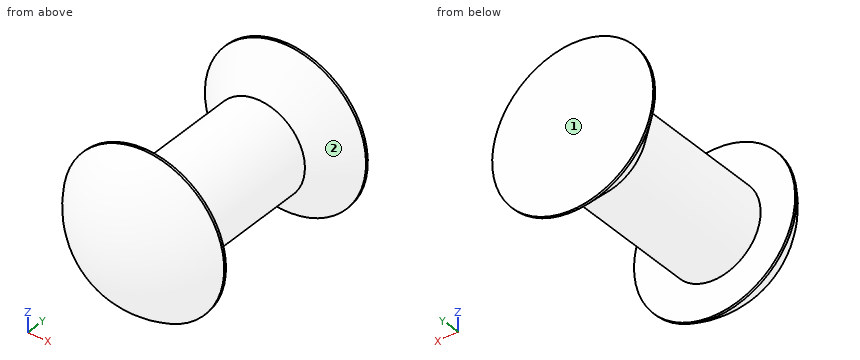
from build123d import *

# Parameters (mm, degrees)
EXTRUDE_1_DEPTH      = 0.4
EXTRUDE_1_DEPTH_BACK = 2
SKETCH_2_R           = 2
SKETCH_3_R           = 3.5
EXTRUDE_2_DEPTH      = 0.1
DOME_1_FACE_RADIUS   = 3.5
DOME_1_HEIGHT        = 2


with BuildPart() as part:
    # Эскиз1 → Revolve 344 (revolve)
    with BuildSketch(Plane.XY, mode=Mode.PRIVATE) as revolve_344_sk:
        with BuildLine():
            Line((0, 0), (1.6, 0))
            ThreePointArc((1.6, 0), (1.882842712, 0.117157288), (2, 0.4))
            Line((2, 0.4), (2, 6))
            Line((2, 6), (3.5, 7.5))
            Line((3.5, 7.5), (3.5, 7.6))
            Line((3.5, 7.6), (0, 7.6))
            Line((0, 7.6), (0, 0))
        make_face()
    revolve(revolve_344_sk.sketch.rotate(Axis((0, 11.283972125, 0), (0, -1, 0)), 90), axis=Axis((0, 11.283972125, 0), (0, -1, 0)))

    # Эскиз2 → Вытянуть1 (add, two sides: drawn at the far end of the back side and taken through both)
    with BuildSketch(Plane.XZ.offset(-EXTRUDE_1_DEPTH_BACK)):
        with Locations(Location((0, 0, 0), (0, 0, 90))):
            Circle(SKETCH_2_R)
    extrude(amount=EXTRUDE_1_DEPTH + EXTRUDE_1_DEPTH_BACK)

    # Эскиз3 → Вытянуть2 (add)
    with BuildSketch(Plane.XZ.offset(0.4)):
        with Locations(Location((0, 0, 0), (0, 0, 90))):
            Circle(SKETCH_3_R)
    extrude(amount=EXTRUDE_2_DEPTH)

    # Купол1: a dome of height H over a round flat face of radius A is a cap of a sphere of radius (A * A + H * H) / (2 * H)
    dome_1_r = (DOME_1_FACE_RADIUS * DOME_1_FACE_RADIUS + DOME_1_HEIGHT * DOME_1_HEIGHT) / (2 * DOME_1_HEIGHT)
    dome_1_base = Plane((0, -0.5, 0), z_dir=(0, -1, 0))
    with Locations(dome_1_base.offset(DOME_1_HEIGHT - dome_1_r)):
        dome_1_ball = Sphere(dome_1_r, mode=Mode.PRIVATE)
    add(split(dome_1_ball, bisect_by=dome_1_base, keep=Keep.TOP, mode=Mode.PRIVATE))


solid = part.part
Geometry check sheet. Reference: the model listing, model coordinates, mm. Face numbers are marked on the shaded views. Give positions to 0.01 mm unless a question says otherwise; leave off trailing zeros. Loops run counter-clockwise (first coordinate to the right, second up) from the corner with the lowest first, then second, coordinate; pieces in that order, holes last.
(1) Section check D-D on y = 1. Record the cut outline in (x, z), then the cut area to 3 significant figures.
From the geometry:
outline: circle Ø4 at (0, 0)
area: 12.6 mm2
(2) Section check C-C on y = 7. Record the cut outline in (x, z).
From the geometry:
outline: circle Ø6 at (0, 0)
(3) Release check for a two-part mould opening along Y. For the marked faces 1 and 2 record: released by +Y, released by -Y, zero draft, split by the parting line, or undercut.
From the geometry:
face 1: released by +Y
face 2: undercut
(4) Depth check by flat-ended pin: pin 1 Ø1 at (y, z) = (3.5, -2) entering from -X; pin 2 Ø3 at (y, z) = (3, -1) entering from +X; pin 3 Ø1.5 at (x, z) = (1.5, 2) entering from -Y. Enter the tip coordinate at first touch or a pass-through.
From the geometry:
pin 1: stops at x = -1.32
pin 2: stops at x = 2
pin 3: stops at y = -2.1
(5) Thickness scan on L1, parallel to Y at x = 1.5, z = -1.25; L2, parallel to Y at x = -1.5, z = 2.75; L3, parallel to Y at x = 2.5, z = -1. Record the ranges inside material, lowest first.
From the geometry:
L1: y = -2 to 7.6
L2: y = -1.02 to -0.4, 7.13 to 7.6
L3: y = -1.48 to -0.4, 6.69 to 7.6
